For this review, take the finished solid that the model builds, in its own axes (mm). A direction names the side the tool comes from. Round coordinates to 2 decimals unless told otherwise and drop trailing zeros. Order: outer loops, then holes, each group sorted by start corner. A loop starts at its lowest first (then second) coordinate and runs counter-clockwise, first axis right, second up. Notation, with made-up numbers: (54.25, -26.5) -> (92.25, -26.5) arc R18 cw to (92.25, -17.5) -> close; hole circle Ø2 at (87.25, 26.5). An arc over 180 degrees is marked (long way). Use a Markdown table: item, result. Add a question column.
1) Consider section A-A (y = 27.5). State the section outline as (x, z) points.
2) Draft analysis for pull direction Y (two halves, no side actions). For faces 1 (the face through (0, -30, 1)), 2 (the face through (-43, -39, 1)), state which applies: pulls with the +Y half, pulls with the -Y half, needs draft (parallel to the pull), parting line crosses it, or undercut.
3) Consider section C-C (x = 7.5). State the section outline as (y, z) points.
4) Clearance check with flat-ended pins moving along their axes: P1, Ø3, axis at x = -24, y = 22, coming from the -Z side; P2, Ø3, axis at x = 29.5, y = 7.5, coming from the +Z side; P3, Ø1.5, axis at y = -13, z = 2, coming from the -X side; P4, Ø1.6, axis at y = -2.5, z = 0.5, coming from the +X side. State where each tip first meets the part, or that it passes through.
5) Consider section B-B (z = 5.5). State the section outline as (x, y) points, plus the area to 3 significant figures.
6) Machinability: for faces 3 (the face through (-15, 0, 1)), 4 (the face through (-39, -30, 1)), 5 (the face through (39, -30, 1)), which of the approach directions +Z, -Z, +X, -X, +Y, -Y give a long, thin tool a straight path to every point of the face, cutting with its end or side? Answer none if there is none.
7) Consider section D-D (y = 9). State the section outline as (x, z) points, plus the area to 3 significant figures.
8) Wall thickness on line 1 along Y through (x, z) = (-22, 1.1); line 2 along Y through (x, z) = (-26, 3.25); line 3 along Y through (x, z) = (-9, 1): over which ranges is each line inside the solid? List them lowest first. Write a range as [from, to].
```python
from build123d import *

# Parameters (mm, degrees)
F0_R     = 3.5
F0_R_2   = 1.5
F0_W     = 30
F0_H     = 60
F1_DEPTH = 2
F0_R_3   = 1.75
F2_DEPTH = 7


with BuildPart() as f1:
    # F0 (on Top) → F1 (new body)
    with BuildSketch(Plane.XY):
        Polygon((43, 30), (43, 48), (35, 48), (-35, 48), (-43, 48), (-43, 30), (-35, 30), (-35, 0), (-35, -30), (-43, -30), (-43, -48), (-35, -48), (35, -48), (43, -48), (43, -30), (35, -30), (35, 0), (35, 30), align=None)
        with Locations((-26, -35)):
            Circle(F0_R, mode=Mode.SUBTRACT)
        with Locations((-22, -9)):
            Circle(F0_R_2, mode=Mode.SUBTRACT)
        with Locations((26, -35)):
            Circle(F0_R, mode=Mode.SUBTRACT)
        with Locations((22, -9)):
            Circle(F0_R_2, mode=Mode.SUBTRACT)
        with Locations((-22, 9)):
            Circle(F0_R_2, mode=Mode.SUBTRACT)
        with Locations((-26, 35)):
            Circle(F0_R, mode=Mode.SUBTRACT)
        Rectangle(F0_W, F0_H, mode=Mode.SUBTRACT)
        with Locations((22, 9)):
            Circle(F0_R_2, mode=Mode.SUBTRACT)
        with Locations((26, 35)):
            Circle(F0_R, mode=Mode.SUBTRACT)
    extrude(amount=F1_DEPTH)

    # F0 (on Top) → F2 (join)
    with BuildSketch(Plane.XY):
        with Locations((-26, 35)):
            Circle(F0_R)
        with Locations((-26, 35)):
            Circle(F0_R_3, mode=Mode.SUBTRACT)
        with Locations((26, 35)):
            Circle(F0_R)
        with Locations((26, 35)):
            Circle(F0_R_3, mode=Mode.SUBTRACT)
        with Locations((26, -35)):
            Circle(F0_R)
        with Locations((26, -35)):
            Circle(F0_R_3, mode=Mode.SUBTRACT)
        with Locations((-26, -35)):
            Circle(F0_R)
        with Locations((-26, -35)):
            Circle(F0_R_3, mode=Mode.SUBTRACT)
    extrude(amount=F2_DEPTH)


solid = f1.part
```
Results list:
| question | item | result |
|---|---|---|
| 1 | outline | (-35, 0) -> (-15, 0) -> (-15, 2) -> (-35, 2) -> close; (15, 0) -> (35, 0) -> (35, 2) -> (15, 2) -> close |
| 2 | face 1 | undercut |
| 2 | face 2 | needs draft |
| 3 | outline | (-48, 0) -> (-30, 0) -> (-30, 2) -> (-48, 2) -> close; (30, 0) -> (48, 0) -> (48, 2) -> (30, 2) -> close |
| 4 | P1 | z = 0 |
| 4 | P2 | z = 2 |
| 4 | P3 | x = -35 |
| 4 | P4 | x = 35 |
| 5 | outline | circle Ø7 at (-26, -35); circle Ø7 at (-26, 35); circle Ø7 at (26, -35); circle Ø7 at (26, 35); hole circle Ø3.5 at (-26, -35); hole circle Ø3.5 at (-26, 35); hole circle Ø3.5 at (26, -35); hole circle Ø3.5 at (26, 35) |
| 5 | area | 115 mm2 |
| 6 | face 3 | +Z, -Z |
| 6 | face 4 | +Z, -Z, -X |
| 6 | face 5 | +Z, -Z, +X |
| 7 | outline | (-35, 0) -> (-23.5, 0) -> (-23.5, 2) -> (-35, 2) -> close; (-20.5, 0) -> (-15, 0) -> (-15, 2) -> (-20.5, 2) -> close; (15, 0) -> (20.5, 0) -> (20.5, 2) -> (15, 2) -> close; (23.5, 0) -> (35, 0) -> (35, 2) -> (23.5, 2) -> close |
| 7 | area | 68.0 mm2 |
| 8 | line 1 | [-48, -10.5], [-7.5, 7.5], [10.5, 48] |
| 8 | line 2 | [-38.5, -36.75], [-33.25, -31.5], [31.5, 33.25], [36.75, 38.5] |
| 8 | line 3 | [-48, -30], [30, 48] |
